from build123d import *

# Parameters (mm, degrees)
SKETCH1_R           = 12
BOSS_EXTRUDE1_DEPTH = 100
BOSS_EXTRUDE2_DEPTH = 12
SKETCH4_OUTSIDE_W   = 131.89
SKETCH4_OUTSIDE_H   = 126.63
SKETCH4_OUTSIDE_R   = 17
CUT_EXTRUDE1_DEPTH  = 12
CUT_EXTRUDE1_DRAFT  = -70
BOSS_EXTRUDE3_START = 1
SKETCH5_R           = 12
BOSS_EXTRUDE3_DEPTH = 1
CHAMFER1_SIZE       = 3


with BuildPart() as part:
    # Sketch1 → Boss-Extrude1 (new body)
    with BuildSketch(Plane(origin=(0, 0, 0), x_dir=(1, 0, 0), z_dir=(0, 1, 0))):
        with Locations(Location((0, 0, 0), (0, 0, 270))):
            Circle(SKETCH1_R)
    extrude(amount=BOSS_EXTRUDE1_DEPTH)

    # Sketch2 → Boss-Extrude2 (add)
    with BuildSketch(Plane(origin=(0, 100, 0), x_dir=(1, 0, 0), z_dir=(0, 1, 0))):
        Polygon((19.629909152, 0), (9.814954576, 17), (-9.814954576, 17), (-19.629909152, 0), (-9.814954576, -17), (9.814954576, -17), align=None)
    extrude(amount=BOSS_EXTRUDE2_DEPTH)


with BuildPart() as cut_extrude1_tool:
    # Sketch4 outside → Cut-Extrude1 (with draft: the straight prism first)
    with BuildSketch(Plane(origin=(0, 112, 0), x_dir=(1, 0, 0), z_dir=(0, 1, 0))):
        Rectangle(SKETCH4_OUTSIDE_W, SKETCH4_OUTSIDE_H)
        Circle(SKETCH4_OUTSIDE_R, mode=Mode.SUBTRACT)
    extrude(amount=-CUT_EXTRUDE1_DEPTH)
    # Cut-Extrude1: the draft: its side faces are tilted about the plane it starts from
    cut_extrude1_sides = [cut_extrude1_tool.faces().sort_by_distance(p)[0] for p in [
        (0, 106, 63.315),
        (65.945, 106, 0),
        (0, 106, -63.315),
        (-65.945, 106, 0),
        (-17, 106, 0),
    ]]
    draft(cut_extrude1_sides, Plane(origin=(0, 112, 0), x_dir=(1, 0, 0), z_dir=(0, 1, 0)), CUT_EXTRUDE1_DRAFT)


with BuildPart() as part_1:
    add(part.part)

    # Cut-Extrude1: cut by cut_extrude1_tool
    add(cut_extrude1_tool.part, mode=Mode.SUBTRACT)

    # Sketch5 → Boss-Extrude3 (add)
    with BuildSketch(Plane.XZ.offset(-100).offset(BOSS_EXTRUDE3_START)):
        with BuildLine():
            ThreePointArc((16.51491761, -4.032058572), (16.878293743, -2.030566501), (17, 0))
            ThreePointArc((17, 0), (16.420739111, 4.399923526), (14.722432113, 8.499999569))
            ThreePointArc((14.722432113, 8.499999569), (8.500000217, 14.722431739), (3e-09, 17))
            ThreePointArc((3e-09, 17), (-8.500000031, 14.722431846), (-14.722431902, 8.499999935))
            ThreePointArc((-14.722431902, 8.499999935), (-17, -1.47e-07), (-14.722431755, -8.50000019))
            ThreePointArc((-14.722431755, -8.50000019), (-8.499999905, -14.722431919), (0, -17))
            ThreePointArc((0, -17), (8.499999905, -14.722431919), (14.722431755, -8.50000019))
            ThreePointArc((14.722431755, -8.50000019), (15.632314361, -6.680624799), (16.318367478, -4.765593652))
            ThreePointArc((16.318367478, -4.765593652), (16.310925004, -4.370499183), (16.51491761, -4.032058572))
        make_face()
        with Locations(Location((0, 0, 0), (0, 0, 270))):
            Circle(SKETCH5_R, mode=Mode.SUBTRACT)
    extrude(amount=-BOSS_EXTRUDE3_DEPTH)

    # Chamfer1
    chamfer1_edges = [part_1.edges().sort_by_distance(p)[0] for p in [
        (0, 0, -12),
    ]]
    chamfer(chamfer1_edges, length=CHAMFER1_SIZE)


solid = part_1.part
Design review of the part built by this model. Coordinates are the model's own, in mm. A direction names the side the tool comes from. Round coordinates to 2 decimals unless told otherwise and drop trailing zeros. Write each loop counter-clockwise with the first axis right and the second up, starting at its lowest first coordinate (ties: lowest second). Pieces come first, ordered by that corner, then holes. Notation, with made-up numbers: (5.5, 36.5) -> (40.5, 36.5) arc R17 cw to (40.5, 40.5) -> close; hole circle Ø8 at (33, 61). An arc over 180 degrees is marked (long way). One line per question, with ' | ' between items.
(1) Take a section at A-A, the plane y = 78. State the section outline as (x, z) points.
Result sheet:
outline: circle Ø24 at (0, 0)
(2) Insertion check: P1, Ø8, axis at y = 15.5, z = 0.5, coming from the -X side; P2, Ø1.5, axis at x = -18, z = -0.5, coming from the -Y side; P3, Ø4, axis at x = 4.5, z = -12, coming from the -Y side. Each pin has a flat end and moves straight along its axis. Give the tip position at first contact, or say it passes through.
Result sheet:
P1: x = -12 | P2: y = 100 | P3: y = 1.82
(3) Draft analysis for pull direction Z (two halves, no side actions). For faces 1 (the cylindrical face through (3.604, 50.328, 11.446)), 2 (the conical face through (-8.78, 111.77, -15.29)), 3 (the flat face through (-14.79, 105.92, 8.38)), state which applies: released by +Z, released by -Z, zero draft, split by the parting line, or undercut.
Result sheet:
face 1: split by the parting line | face 2: released by -Z | face 3: released by +Z
(4) Machinability: for faces 4 (the flat face through (9, 100, -15)), 5 (the flat face through (4, 99, 12)), 6 (the flat face through (14.654, 105.916, 8.619)), 7 (the flat face through (-8.5, 100, 15.2)), 8 (the flat face through (18, 100, 0)), which of the approach directions +Z, -Z, +X, -X, +Y, -Y give a long, thin tool a straight path to every point of the face, cutting with its end or side? Answer none if there is none.
Result sheet:
face 4: -Z, +X, -Y | face 5: -Y | face 6: +Z, +X, +Y, -Y | face 7: +Z, -X, -Y | face 8: +X, -Y
(5) Wall thickness on line 1 (Y direction, x = 11, z = 10.5); line 2 (Z direction, x = -10, y = 94); line 3 (Z direction, x = 0.5, y = 50): over which ranges is each line inside the solid? List them lowest first. Write a range as [from, to].
Result sheet:
line 1: [99, 112] | line 2: [-6.63, 6.63] | line 3: [-11.99, 11.99]
